Design review of the part built by this model. Coordinates are the model's own, in mm. Face numbers are marked on the shaded views. A direction names the side the tool comes from. Coordinates: 2 decimals unless noted, no trailing zeros. Write each loop counter-clockwise with the first axis right and the second up, starting at its lowest first coordinate (ties: lowest second). Pieces come first, ordered by that corner, then holes. Notation, with made-up numbers: M 38.25,78.25 L 74.25,78.25 A31 ccw 74.25,102.25 Z; hole C -4.5,62.25 d10. An arc over 180 degrees is marked long. One line per question, with ' | ' between items.
from build123d import *

# Parameters (mm, degrees)
SKETCH_1_W      = 32
SKETCH_1_H      = 32
SKETCH_1_R      = 1
EXTRUDE_1_DEPTH = 1.5
SKETCH_2_W      = 18
SKETCH_2_H      = 18
SKETCH_2_R      = 6
EXTRUDE_2_DEPTH = 9.5


with BuildPart() as part:
    # ｽｹｯﾁ1 → ﾎﾞｽ - 押し出し1 (new body)
    with BuildSketch(Plane.XY):
        Rectangle(SKETCH_1_W, SKETCH_1_H)
        with Locations((-14, 14)):
            Circle(SKETCH_1_R, mode=Mode.SUBTRACT)
        with Locations((14, 14)):
            Circle(SKETCH_1_R, mode=Mode.SUBTRACT)
        with Locations((14, -14)):
            Circle(SKETCH_1_R, mode=Mode.SUBTRACT)
        with Locations((-14, -14)):
            Circle(SKETCH_1_R, mode=Mode.SUBTRACT)
    extrude(amount=EXTRUDE_1_DEPTH)

    # ｽｹｯﾁ2 → ﾎﾞｽ - 押し出し2 (add)
    with BuildSketch(Plane.XY.offset(1.5)):
        Rectangle(SKETCH_2_W, SKETCH_2_H)
        Circle(SKETCH_2_R, mode=Mode.SUBTRACT)
    extrude(amount=EXTRUDE_2_DEPTH)


solid = part.part
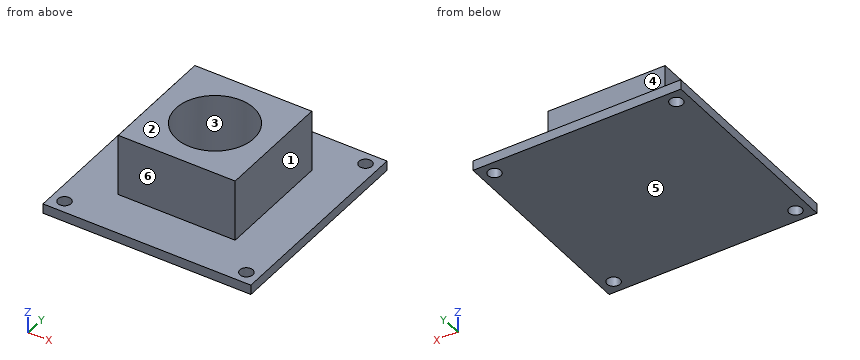
1. Take a section at A-A (x = -14). Write out the cut boundary in (y, z), then the cut area to 3 significant figures.
Answer sheet:
outline: M -16,0 L -15,0 L -15,1.5 L -16,1.5 Z; M -13,0 L 13,0 L 13,1.5 L -13,1.5 Z; M 15,0 L 16,0 L 16,1.5 L 15,1.5 Z | area: 42.0 mm^2
2. Tool access review of the marked faces 4, 5 and 6: name each direction out of +Z, -Z, +X, -X, +Y, -Y from which nothing blocks a thin tool from reaching the whole face with its end or side.
Answer sheet:
face 4: +Z, +X, -X, +Y | face 5: -Z, +X, -X, +Y, -Y | face 6: +Z, +X, -X, -Y
3. Insertion check: pin 1 Ø4 at (x, y) = (10, 12) entering from +Z; pin 2 Ø1 at (y, z) = (-2.5, 6.5) entering from -X; pin 3 Ø4 at (x, z) = (8.5, 5) entering from +Y. Each pin has a flat end and moves straight along its axis. Give the tip position at first contact, or say it passes through.
Answer sheet:
pin 1: z = 1.5 | pin 2: x = -9 | pin 3: y = 9
4. Take a section at C-C (z = 6). Write out the cut boundary in (x, y).
Answer sheet:
outline: M -9,-9 L 9,-9 L 9,9 L -9,9 Z; hole C 0,0 d12
5. Draft analysis for pull direction X (two halves, no side actions). For the marked faces 1, 2 and 3, state which applies: pulls with the +X half, pulls with the -X half, needs draft (parallel to the pull), parting line crosses it, or undercut.
Answer sheet:
face 1: pulls with the +X half | face 2: needs draft | face 3: undercut
6. Take a section at D-D (y = 0). Write out the cut boundary in (x, z).
Answer sheet:
outline: M -16,0 L 16,0 L 16,1.5 L 9,1.5 L 9,11 L 6,11 L 6,1.5 L -6,1.5 L -6,11 L -9,11 L -9,1.5 L -16,1.5 Z
7. To check wall thickness, follow line 1 along Z through (x, y) = (-9, 14.5); line 2 along X through (y, z) = (-3.5, 2.75); line 3 along Y through (x, z) = (6.5, 9.25). State the ranges of each line that lie inside material, in increasing order. Write a range as [from, to].
Answer sheet:
line 1: [0, 1.5] | line 2: [-9, -4.87], [4.87, 9] | line 3: [-9, 9]
